Design review of the part shown in the three views and the two pictorial views. Dimensions are in mm from the part's minimum x, y and z. A direction names the side the tool comes from. Give positions to 0.01 mm unless a question says otherwise; leave off trailing zeros. Order: outer loops, then holes, each group sorted by start corner. A loop starts at its lowest first (then second) coordinate and runs counter-clockwise, first axis right, second up. Notation, with made-up numbers: (50, 86.25) -> (93, 86.25) arc R16 cw to (93, 91.25) -> close; hole circle Ø9 at (-24, 4.5). An arc over 180 degrees is marked (long way). Answer in a Markdown table with one row per item. Add a question column.
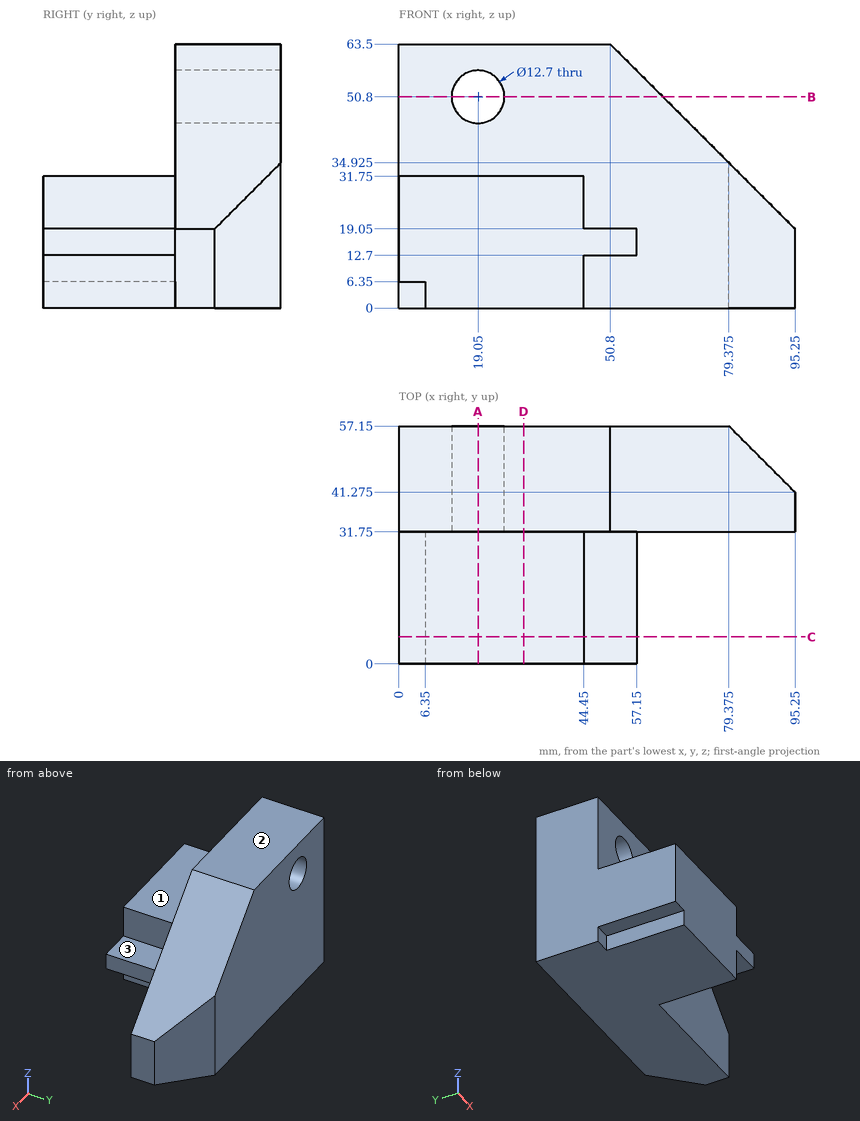
1) Machinability: for the marked faces 1, 2 and 3, which of the approach directions +Z, -Z, +X, -X, +Y, -Y give a long, thin tool a straight path to every point of the face, cutting with its end or side? Answer none if there is none.
2) Add section A-A, the plane x = 19.05. Write out the cut boundary in (y, z), and give its area (3 significant figures).
3) For L1, parallel to Z at x = 19.05, y = 49.5; L2, parallel to Z at x = 16, y = 2.5; L3, parallel to X at y = 10.5, z = 3.5, list the stretches that pass through material, from the lowest coordinate up.
4) Clearance check with flat-ended pins moving along their axes: P1, Ø14, axis at x = 50, y = 20, coming from the +Z side; P2, Ø4, axis at y = 9.5, z = 25, coming from the +X side; P3, Ø3, axis at x = 4, y = 12, coming from the -Z side. State where each tip first meets the part, or that it passes through.
5) Add section B-B, the plane z = 50.8. Write out the cut boundary in (x, y).
6) Add section C-C, the plane y = 6.5. Write out the cut boundary in (x, z), and give its area (3 significant figures).
7) Add section D-D, the plane x = 30. Write out the cut boundary in (y, z), and give its area (3 significant figures).
Verdict:
| question | item | result |
|---|---|---|
| 1 | face 1 | +Z, +X, -X, -Y |
| 1 | face 2 | +Z, +X, -X, +Y, -Y |
| 1 | face 3 | +Z, +X, -Y |
| 2 | outline | (0, 0) -> (57.15, 0) -> (57.15, 44.45) -> (31.75, 44.45) -> (31.75, 31.75) -> (0, 31.75) -> close; (31.75, 57.15) -> (57.15, 57.15) -> (57.15, 63.5) -> (31.75, 63.5) -> close |
| 2 | area | 2,300 mm2 |
| 3 | L1 | z = 0 to 44.45, 57.15 to 63.5 |
| 3 | L2 | z = 0 to 31.75 |
| 3 | L3 | x = 6.35 to 44.45 |
| 4 | P1 | stops at z = 31.75 |
| 4 | P2 | stops at x = 44.45 |
| 4 | P3 | stops at z = 6.35 |
| 5 | outline | (0, 31.75) -> (12.7, 31.75) -> (12.7, 57.15) -> (0, 57.15) -> close; (25.4, 31.75) -> (63.5, 31.75) -> (63.5, 57.15) -> (25.4, 57.15) -> close |
| 6 | outline | (0, 6.35) -> (6.35, 6.35) -> (6.35, 0) -> (44.45, 0) -> (44.45, 12.7) -> (57.15, 12.7) -> (57.15, 19.05) -> (44.45, 19.05) -> (44.45, 31.75) -> (0, 31.75) -> close |
| 6 | area | 1,450 mm2 |
| 7 | outline | (0, 0) -> (57.15, 0) -> (57.15, 63.5) -> (31.75, 63.5) -> (31.75, 31.75) -> (0, 31.75) -> close |
| 7 | area | 2,620 mm2 |
